Source: CAD feature listing. Evaluate the final solid. Frame: model axes, mm. Face numbers are marked on the shaded views. A direction names the side the tool comes from. Coordinates: 2 decimals unless noted, no trailing zeros. Order: outer loops, then holes, each group sorted by start corner. A loop starts at its lowest first (then second) coordinate and runs counter-clockwise, first axis right, second up.
Item 1: Contact query for flat-ended pins moving along their axis: P1, Ø6, axis at x = -24.5, z = -29.5, coming from the -Y side; P2, Ø6, axis at x = -6.5, y = 27.5, coming from the +Z side; P3, Ø3.5, axis at x = -9, z = -36, coming from the +Y side. Output: stop coordinate, or through.
Item 2: Section A-A on y = 13. Return the cut outline in (x, z), then the cut area to 3 significant figures.
Item 3: Section C-C on z = -22.86. Return the cut outline in (x, y), then the cut area to 3 significant figures.
Item 4: Reachability of the marked faces 1 and 2 from +Z, -Z, +X, -X, +Y, -Y: full face, straight path, thin tool, end or side. Return the list, or none.
Item 5: Section D-D on y = 30. Return the cut outline in (x, z), then the cut area to 3 significant figures.
Item 6: Ray query, line 1 (X direction, y = 24, z = -40); line 2 (X direction, y = 21, z = -31.75); line 3 (X direction, y = 22.5, z = -31). Return the intervals inside material, ascending.
Item 7: Mould query, pull axis Z, two halves, no side actions, for the marked faces 3, 4, 5 and 6. Classes: released by +Z, released by -Z, zero draft, split by the parting line, or undercut.
Item 8: Section B-B on z = -31.75. Return the cut outline in (x, y).
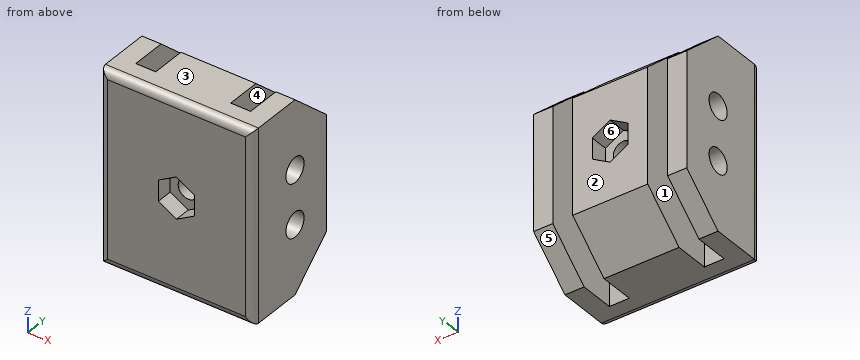
from build123d import *

# Parameters (mm, degrees)
SKETCH1_W           = 63.5
SKETCH1_H           = 6.35
BOSS_EXTRUDE1_DEPTH = 50.8
BOSS_EXTRUDE2_DEPTH = 50.8
SKETCH10_W          = 6.604
SKETCH10_H          = 25.629031657
CUT_EXTRUDE1_DEPTH  = 88.854357354
LPATTERN3_COUNT     = 2
LPATTERN3_PITCH     = 31.496
SKETCH11_R          = 4.09575
CUT_EXTRUDE2_DEPTH  = 88.854357354
CUT_EXTRUDE3_DEPTH  = 5.953125
LPATTERN4_COUNT     = 2
LPATTERN4_PITCH     = 27.94
SKETCH20_R          = 3.302
CUT_EXTRUDE4_DEPTH  = 21.986875
FILLET1_R           = 2.54


with BuildPart() as part:
    # Sketch1 → Boss-Extrude1 (new body)
    with BuildSketch(Plane(origin=(0, 0, 0), x_dir=(0, 0, -1), z_dir=(1, 0, 0))):
        with Locations((31.75, 3.175)):
            Rectangle(SKETCH1_W, SKETCH1_H)
    extrude(amount=-BOSS_EXTRUDE1_DEPTH)

    # Sketch2 → Boss-Extrude2 (add)
    with BuildSketch(Plane(origin=(0, 0, 0), x_dir=(0, 0, -1), z_dir=(1, 0, 0))):
        Polygon((0, 6.35), (0, 19.05), (12.7, 33.249031657), (50.8, 33.249031657), (63.5, 19.05), (63.5, 6.35), align=None)
    extrude(amount=-BOSS_EXTRUDE2_DEPTH)

    # Sketch10 → Cut-Extrude1 (cut, through all)
    with BuildSketch(Plane(origin=(0, 0, -63.5), x_dir=(-1, 0, 0), z_dir=(0, 0, -1))):
        with Locations((9.652, 20.434515829)):
            Rectangle(SKETCH10_W, SKETCH10_H)
    cut_extrude1 = extrude(amount=-CUT_EXTRUDE1_DEPTH, mode=Mode.SUBTRACT)

    # LPattern3: Cut-Extrude1 ×2
    with Locations(*[(-i * LPATTERN3_PITCH, 0, 0) for i in range(1, LPATTERN3_COUNT)]):
        add(cut_extrude1, mode=Mode.SUBTRACT)

    # Sketch11 → Cut-Extrude2 (cut, through all)
    with BuildSketch(Plane(origin=(0, 0, 0), x_dir=(0, 0, -1), z_dir=(1, 0, 0))):
        with Locations((22.86, 19.05)):
            Circle(SKETCH11_R)
        with Locations((40.64, 19.05)):
            Circle(SKETCH11_R)
    extrude(amount=-CUT_EXTRUDE2_DEPTH, mode=Mode.SUBTRACT)

    # Sketch19 → Cut-Extrude3 (cut)
    with BuildSketch(Plane(origin=(0, 33.249031657, 0), x_dir=(1, 0, 0), z_dir=(0, 1, 0))):
        Polygon((-19.448913651, 35.185861306), (-25.4, 38.621722611), (-31.351086349, 35.185861306), (-31.351086349, 28.314138694), (-25.4, 24.878277389), (-19.448913651, 28.314138694), align=None)
    cut_extrude3 = extrude(amount=-CUT_EXTRUDE3_DEPTH, mode=Mode.SUBTRACT)

    # LPattern4: Cut-Extrude3 ×2
    with Locations(*[(0, -i * LPATTERN4_PITCH, 0) for i in range(1, LPATTERN4_COUNT)]):
        add(cut_extrude3, mode=Mode.SUBTRACT)

    # Sketch20 → Cut-Extrude4 (cut)
    with BuildSketch(Plane(origin=(0, 27.295906657, 0), x_dir=(1, 0, 0), z_dir=(0, 1, 0))):
        with Locations(Location((-25.4, 31.75, 0), (0, 0, 270))):
            Circle(SKETCH20_R)
    extrude(amount=-CUT_EXTRUDE4_DEPTH, mode=Mode.SUBTRACT)

    # Fillet1
    fillet1_edges = [part.edges().sort_by_distance(p)[0] for p in [
        (0, 0, -31.75),
        (-50.8, 0, -31.75),
        (-25.4, 0, -63.5),
        (-25.4, 0, 0),
    ]]
    fillet(fillet1_edges, radius=FILLET1_R)


solid = part.part
Answer list:
1. P1: stops at y = 5.31
1. P2: stops at z = -4.88
1. P3: stops at y = 7.62
2. outline: (-50.8, -63.5) - (-44.45, -63.5) - (-44.45, 0) - (-50.8, 0) - close; (-37.85, -63.5) - (-12.95, -63.5) - (-12.95, 0) - (-37.85, 0) - close; (-6.35, -63.5) - (0, -63.5) - (0, 0) - (-6.35, 0) - close; hole circle Ø6.6 at (-25.4, -31.75)
2. area: 2,350 mm2
3. outline: (-50.8, 2.54) arc R2.54 ccw to (-48.26, 0) - (-2.54, 0) arc R2.54 ccw to (0, 2.54) - (0, 14.95) - (-6.35, 14.95) - (-6.35, 7.62) - (-12.95, 7.62) - (-12.95, 14.95) - (-37.85, 14.95) - (-37.85, 7.62) - (-44.45, 7.62) - (-44.45, 14.95) - (-50.8, 14.95) - close; (-50.8, 23.15) - (-44.45, 23.15) - (-44.45, 33.25) - (-50.8, 33.25) - close; (-37.85, 23.15) - (-12.95, 23.15) - (-12.95, 33.25) - (-37.85, 33.25) - close; (-6.35, 23.15) - (0, 23.15) - (0, 33.25) - (-6.35, 33.25) - close
3. area: 1,040 mm2
4. face 1: +Z, -Z, +Y
4. face 2: +Z, -Z, +X, -X, +Y
5. outline: (-50.8, -53.71) - (-44.45, -53.71) - (-44.45, -9.79) - (-50.8, -9.79) - close; (-37.85, -53.71) - (-12.95, -53.71) - (-12.95, -9.79) - (-37.85, -9.79) - close; (-6.35, -53.71) - (0, -53.71) - (0, -9.79) - (-6.35, -9.79) - close; hole (-31.35, -35.19) - (-25.4, -38.62) - (-19.45, -35.19) - (-19.45, -28.31) - (-25.4, -24.88) - (-31.35, -28.31) - close
5. area: 1,530 mm2
6. line 1: x = -50.8 to -44.45, -37.85 to -12.95, -6.35 to 0
6. line 2: x = -50.8 to -44.45, -37.85 to -28.7, -22.1 to -12.95, -6.35 to 0
6. line 3: x = -50.8 to -44.45, -37.85 to -28.62, -22.18 to -12.95, -6.35 to 0
7. face 3: released by +Z
7. face 4: zero draft
7. face 5: released by -Z
7. face 6: undercut
8. outline: (-50.8, 2.54) arc R2.54 ccw to (-48.26, 0) - (-31.35, 0) - (-31.35, 5.31) - (-28.7, 5.31) - (-28.7, 27.3) - (-31.35, 27.3) - (-31.35, 33.25) - (-37.85, 33.25) - (-37.85, 7.62) - (-44.45, 7.62) - (-44.45, 33.25) - (-50.8, 33.25) - close; (-22.1, 5.31) - (-19.45, 5.31) - (-19.45, 0) - (-2.54, 0) arc R2.54 ccw to (0, 2.54) - (0, 33.25) - (-6.35, 33.25) - (-6.35, 7.62) - (-12.95, 7.62) - (-12.95, 33.25) - (-19.45, 33.25) - (-19.45, 27.3) - (-22.1, 27.3) - close
